Part model, mm, in its own coordinate system. Face numbers are marked on the shaded views. Give positions to 0.01 mm unless a question says otherwise; leave off trailing zeros. Write each loop counter-clockwise with the first axis right and the second up, starting at its lowest first coordinate (ties: lowest second). Pieces come first, ordered by that corner, then holes. Notation, with made-up numbers: (25.5, 76) - (61.5, 76) arc R30 ccw to (61.5, 98) - close; hole circle Ø4 at (30, 50). An arc over 180 degrees is marked (long way). Answer in a Markdown table with one row per item. Add a question column.
1. Band-saw the part on C-C on z = 7. Write the cut outline in (x, y) (1 decimal), plus the area to 3 significant figures.
2. Drop flat-ended pins along their axis: pin 1 Ø5 at (x, y) = (-8.5, 8.5) entering from -Z; pin 2 Ø10 at (x, z) = (-24, -4) entering from +Y; pin 3 Ø2.5 at (y, z) = (15, 0.5) entering from -X. Give the stop position or say it passes through.
3. Probe line 1 along X through (y, z) = (-2.8, 0); line 2 along Y through (x, z) = (-1, 9) (3 decimals); line 3 along Y through (x, z) = (-40.5, 5) (3 decimals). List the from-to ranges inside material, lowest first.
4. Band-saw the part on A-A on x = -8. Write the cut outline in (y, z) (1 decimal).
5. Band-saw the part on B-B on z = 0. Write the cut outline in (x, y) (1 decimal), plus the area to 3 significant figures.
6. Pull direction X, two halves, no side cores. Call the marked faces 1, 2 and 3: released by +X, released by -X, zero draft, split by the parting line, or undercut.
7. Band-saw the part on D-D on x = 0. Write the cut outline in (y, z) (1 decimal), plus the area to 3 significant figures.
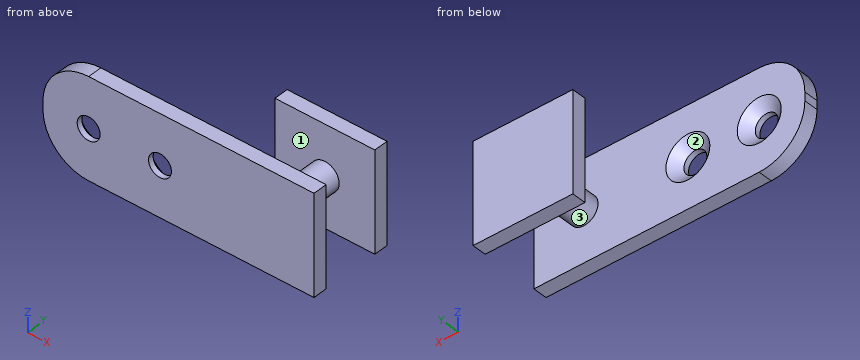
```python
from build123d import *

# Parameters (mm, degrees)
SKETCH1_R                                  = 3.175
BOSS_EXTRUDE1_DEPTH                        = 12.7
SKETCH2_W                                  = 22.225
SKETCH2_H                                  = 22.225
BOSS_EXTRUDE2_DEPTH                        = 3.175
BOSS_EXTRUDE3_DEPTH                        = 3.175
CSK_FOR_10_FLAT_HEAD_MACHINE_SCREW_2_COUNT = 2
CSK_FOR_10_FLAT_HEAD_MACHINE_SCREW_2_PITCH = 15.875


with BuildPart() as part:
    # Sketch1 → Boss-Extrude1 (new body)
    with BuildSketch(Plane(origin=(0, 0, 0), x_dir=(1, 0, 0), z_dir=(0, 1, 0))):
        Circle(SKETCH1_R)
    extrude(amount=BOSS_EXTRUDE1_DEPTH)

    # Sketch2 → Boss-Extrude2 (add)
    with BuildSketch(Plane(origin=(0, 12.7, 0), x_dir=(1, 0, 0), z_dir=(0, 1, 0))):
        Rectangle(SKETCH2_W, SKETCH2_H)
    boss_extrude2 = extrude(amount=BOSS_EXTRUDE2_DEPTH)

    # Mirror1: Boss-Extrude2 across plane
    add(boss_extrude2.mirror(Plane(origin=(0, 6.35, 0), x_dir=(0, 0, 1), z_dir=(0, -1, 0))))

    # Sketch3 → Boss-Extrude3 (add)
    with BuildSketch(Plane.XZ.offset(3.175)):
        with BuildLine():
            Line((-11.1125, -11.1125), (-39.0525, -11.1125))
            ThreePointArc((-39.0525, -11.1125), (-46.236704897, -8.136704897), (-49.2125, -0.9525))
            Line((-49.2125, -0.9525), (-49.2125, 0.9525))
            ThreePointArc((-49.2125, 0.9525), (-46.236704897, 8.136704897), (-39.0525, 11.1125))
            Line((-39.0525, 11.1125), (-11.1125, 11.1125))
            Line((-11.1125, 11.1125), (-11.1125, -11.1125))
        make_face()
    extrude(amount=-BOSS_EXTRUDE3_DEPTH)

    # Sketch6 → CSK for #10 Flat Head Machine Screw (100)1 (revolve, cut)
    with BuildSketch(Plane(origin=(-39.0525, 0, 0), x_dir=(0, 0, 1), z_dir=(1, 0, 0))):
        Polygon((0, 0), (0, 3.175), (2.5527, 3.175), (2.5527, 1.960808018), (4.8895, 0), align=None)
    csk_for_10_flat_head_machine_screw_100 = revolve(axis=Axis((-39.0525, 6.35, 0), (0, -1, 0)), mode=Mode.SUBTRACT)

    # CSK for _10 Flat Head Machine Screw  2: CSK for #10 Flat Head Machine Screw (100)1 ×2
    with Locations(*[(i * CSK_FOR_10_FLAT_HEAD_MACHINE_SCREW_2_PITCH, 0, 0) for i in range(1, CSK_FOR_10_FLAT_HEAD_MACHINE_SCREW_2_COUNT)]):
        add(csk_for_10_flat_head_machine_screw_100, mode=Mode.SUBTRACT)


solid = part.part
```
Values:
| question | item | result |
|---|---|---|
| 1 | outline | (-47.2, -3.2) - (11.1, -3.2) - (11.1, 0) - (-47.2, 0) - close; (-11.1, 12.7) - (11.1, 12.7) - (11.1, 15.9) - (-11.1, 15.9) - close |
| 1 | area | 256 mm² |
| 2 | pin 1 | passes through |
| 2 | pin 2 | stops at y = 0 |
| 2 | pin 3 | stops at x = -11.11 |
| 3 | line 1 | x = -49.21 to -41.61, -36.5 to -25.73, -20.62 to 11.11 |
| 3 | line 2 | y = -3.175 to 0, 12.7 to 15.875 |
| 3 | line 3 | y = -3.175 to 0 |
| 4 | outline | (-3.2, -11.1) - (0, -11.1) - (0, 11.1) - (-3.2, 11.1) - close; (12.7, -11.1) - (15.9, -11.1) - (15.9, 11.1) - (12.7, 11.1) - close |
| 5 | outline | (-49.2, -3.2) - (-41.6, -3.2) - (-41.6, -2) - (-43.9, 0) - (-49.2, 0) - close; (-36.5, -3.2) - (-25.7, -3.2) - (-25.7, -2) - (-28.1, 0) - (-34.2, 0) - (-36.5, -2) - close; (-20.6, -3.2) - (11.1, -3.2) - (11.1, 0) - (3.2, 0) - (3.2, 12.7) - (11.1, 12.7) - (11.1, 15.9) - (-11.1, 15.9) - (-11.1, 12.7) - (-3.2, 12.7) - (-3.2, 0) - (-18.3, 0) - (-20.6, -2) - close |
| 5 | area | 301 mm² |
| 6 | face 1 | zero draft |
| 6 | face 2 | undercut |
| 6 | face 3 | split by the parting line |
| 7 | outline | (-3.2, -11.1) - (0, -11.1) - (0, -3.2) - (12.7, -3.2) - (12.7, -11.1) - (15.9, -11.1) - (15.9, 11.1) - (12.7, 11.1) - (12.7, 3.2) - (0, 3.2) - (0, 11.1) - (-3.2, 11.1) - close |
| 7 | area | 222 mm² |
